Check sheet for the modelled part. Datum: model origin and axes. Units: mm. A direction names the side the tool comes from. Give positions to 0.01 mm unless a question says otherwise; leave off trailing zeros. Loops run counter-clockwise (first coordinate to the right, second up) from the corner with the lowest first, then second, coordinate; pieces in that order, holes last. Notation, with made-up numbers: (89.25, 89) - (147.25, 89) arc R18 cw to (147.25, 113) - close; hole circle Ø2 at (7.25, -39). An arc over 180 degrees is marked (long way). Answer in a Markdown table with one row per item. Add a question column.
(1) Thickness scan on L1, parallel to X at y = 4.5, z = 20; L2, parallel to X at y = 71, z = -13; L3, parallel to X at y = 4, z = -20. Record the ranges inside material, lowest first.
(2) Draft check along X on faces 1 (the face through (-82.21, 2.35, -29.21)), 2 (the face through (-85.24, 89.88, 1.08)), 3 (the face through (76.5, 49, 0)). Enter one of: released by +X, released by -X, zero draft, split by the parting line, or undercut.
(3) Sectioned sample at C-C on z = -20. State how many separate pieces and enclosed holes the cut face has, then the cut area to 3 significant figures.
(4) Sectioned sample at B-B on x = 38. Enter the section's corners in (y, z).
(5) Set-up check for faces 4 (the face through (-76.5, 59, 0)), 5 (the face through (75.62, 8.969, 28.764)), 6 (the face through (76.819, 106.312, -0.623)), 7 (the face through (-78.47, 90.95, 0.78)): record each of +Z, -Z, +X, -X, +Y, -Y from which the full face is reachable in a straight line by a thin tool's end or side.
(6) Go/stop test with flat-tipped pins: P1, Ø5.5, axis at x = 0, z = 20, coming from the -Y side; P2, Ø5, axis at x = -63, z = 19.5, coming from the +Y side; P3, Ø12, axis at y = 85, z = 0, coming from the -X side; P4, Ø1.8, axis at y = 85, z = -15, coming from the +X side. Record where each tip stops, or that it passes through.
(7) Sectioned sample at A-A on y = 44. Enter the section's corners in (x, z).
from build123d import *

# Parameters (mm, degrees)
SKETCH1_W           = 169
SKETCH1_H           = 60
BOSS_EXTRUDE1_DEPTH = 8
SKETCH2_W           = 8
SKETCH2_H           = 60
BOSS_EXTRUDE2_DEPTH = 100
SKETCH3_R           = 10
SKETCH3_R_2         = 1.5
CUT_EXTRUDE1_DEPTH  = 12
SKETCH5_R           = 5
BOSS_EXTRUDE3_DEPTH = 1.5
SKETCH6_R           = 4
CUT_EXTRUDE3_DEPTH  = 15
SKETCH7_R           = 6
CUT_EXTRUDE4_DEPTH  = 4
FILLET1_RADIUS      = 30
FILLET1_LENGTH      = 8
FILLET2_RADIUS      = 30
FILLET2_LENGTH      = 8
FILLET3_R           = 5
FILLET4_R           = 5
FILLET5_R           = 5
FILLET6_R           = 5
CHAMFER1_SIZE       = 2
SKETCH8_R           = 3.1
SKETCH8_R_2         = 3.2
CUT_EXTRUDE5_DEPTH  = 10


with BuildPart() as part:
    # Sketch1 → Boss-Extrude1 (new body)
    with BuildSketch(Plane(origin=(0, 0, 0), x_dir=(1, 0, 0), z_dir=(0, 1, 0))):
        Rectangle(SKETCH1_W, SKETCH1_H)
    extrude(amount=BOSS_EXTRUDE1_DEPTH)

    # Sketch2 → Boss-Extrude2 (add)
    with BuildSketch(Plane(origin=(0, 8, 0), x_dir=(1, 0, 0), z_dir=(0, 1, 0))):
        with Locations((-80.5, 0)):
            Rectangle(SKETCH2_W, SKETCH2_H)
        with Locations((80.5, 0)):
            Rectangle(SKETCH2_W, SKETCH2_H)
    extrude(amount=BOSS_EXTRUDE2_DEPTH)

    # Sketch3 → Cut-Extrude1 (cut)
    with BuildSketch(Plane(origin=(84.5, 0, 0), x_dir=(0, 0, -1), z_dir=(1, 0, 0))):
        with Locations((0, 85)):
            Circle(SKETCH3_R)
        with Locations((0, 70)):
            Circle(SKETCH3_R_2)
        with Locations((0, 100)):
            Circle(SKETCH3_R_2)
        with Locations((-15, 85)):
            Circle(SKETCH3_R_2)
        with Locations((15, 85)):
            Circle(SKETCH3_R_2)
    extrude(amount=-CUT_EXTRUDE1_DEPTH, mode=Mode.SUBTRACT)

    # Sketch5 → Boss-Extrude3 (add)
    with BuildSketch(Plane.ZY.offset(84.5)):
        with Locations(Location((0, 85, 0), (0, 0, 180))):
            Circle(SKETCH5_R)
    extrude(amount=BOSS_EXTRUDE3_DEPTH)

    # Sketch6 → Cut-Extrude3 (cut)
    with BuildSketch(Plane.ZY.offset(86)):
        with Locations((0, 85)):
            Circle(SKETCH6_R)
    extrude(amount=-CUT_EXTRUDE3_DEPTH, mode=Mode.SUBTRACT)

    # Sketch7 → Cut-Extrude4 (cut)
    with BuildSketch(Plane(origin=(-76.5, 0, 0), x_dir=(0, 0, -1), z_dir=(1, 0, 0))):
        with Locations((0, 85)):
            Circle(SKETCH7_R)
    extrude(amount=-CUT_EXTRUDE4_DEPTH, mode=Mode.SUBTRACT)

    # Fillet1: full round fillet: the end face becomes a half cylinder, R = half its width
    fillet1_face = Plane((80.5, 108, 0), x_dir=(-1, 0, 0), z_dir=(0, 1, 0))  # on the end face: x along it, z out of the body
    fillet1_slab = fillet1_face.offset(-FILLET1_RADIUS / 2) * Box(FILLET1_LENGTH, 2 * FILLET1_RADIUS, FILLET1_RADIUS, mode=Mode.PRIVATE)  # the body's end, R deep
    fillet1_round = Plane((80.5, 78, 0), x_dir=(0, 1, 0), z_dir=(-1, 0, 0)) * Cylinder(FILLET1_RADIUS, FILLET1_LENGTH, mode=Mode.PRIVATE)  # its axis R under the face
    add(fillet1_slab - fillet1_round, mode=Mode.SUBTRACT)

    # Fillet2: full round fillet: the end face becomes a half cylinder, R = half its width
    fillet2_face = Plane((-80.5, 108, 0), x_dir=(1, 0, 0), z_dir=(0, 1, 0))  # on the end face: x along it, z out of the body
    fillet2_slab = fillet2_face.offset(-FILLET2_RADIUS / 2) * Box(FILLET2_LENGTH, 2 * FILLET2_RADIUS, FILLET2_RADIUS, mode=Mode.PRIVATE)  # the body's end, R deep
    fillet2_round = Plane((-80.5, 78, 0), x_dir=(0, 1, 0), z_dir=(1, 0, 0)) * Cylinder(FILLET2_RADIUS, FILLET2_LENGTH, mode=Mode.PRIVATE)  # its axis R under the face
    add(fillet2_slab - fillet2_round, mode=Mode.SUBTRACT)

    # Fillet3
    fillet3_edges = [part.edges().sort_by_distance(p)[0] for p in [
        (76.5, 8, 0),
    ]]
    fillet(fillet3_edges, radius=FILLET3_R)

    # Fillet4
    fillet4_edges = [part.edges().sort_by_distance(p)[0] for p in [
        (-76.5, 8, 0),
    ]]
    fillet(fillet4_edges, radius=FILLET4_R)

    # Fillet5
    fillet5_edges = [part.edges().sort_by_distance(p)[0] for p in [
        (84.5, 0, 0),
    ]]
    fillet(fillet5_edges, radius=FILLET5_R)

    # Fillet6
    fillet6_edges = [part.edges().sort_by_distance(p)[0] for p in [
        (-84.5, 0, 0),
    ]]
    fillet(fillet6_edges, radius=FILLET6_R)

    # Chamfer1
    chamfer1_edges = [part.edges().sort_by_distance(p)[0] for p in [
        (75.035533906, 9.464466094, -30),
        (75.035533906, 9.464466094, 30),
        (0, 8, 30),
        (-75.035533906, 9.464466094, 30),
        (-75.035533906, 9.464466094, -30),
        (0, 0, -30),
        (83.035533906, 1.464466094, 30),
        (83.035533906, 1.464466094, -30),
        (0, 0, 30),
        (-83.035533906, 1.464466094, -30),
        (-83.035533906, 1.464466094, 30),
        (76.5, 45.5, -30),
        (84.5, 41.5, -30),
        (84.5, 41.5, 30),
        (76.5, 45.5, 30),
        (76.5, 108, 0),
        (84.5, 108, 0),
        (-84.5, 41.5, -30),
        (-76.5, 45.5, -30),
        (-76.5, 45.5, 30),
        (-84.5, 41.5, 30),
        (-84.5, 108, 0),
        (-76.5, 108, 0),
        (0, 8, -30),
    ]]
    chamfer(chamfer1_edges, length=CHAMFER1_SIZE)

    # Sketch8 → Cut-Extrude5 (cut)
    with BuildSketch(Plane(origin=(0, 8, 0), x_dir=(1, 0, 0), z_dir=(0, 1, 0))):
        with Locations(Location((0, 0, 0), (0, 0, 270))):
            Circle(SKETCH8_R)
        with Locations(Location((0, 20, 0), (0, 0, 270))):
            Circle(SKETCH8_R)
        with Locations(Location((0, -20, 0), (0, 0, 270))):
            Circle(SKETCH8_R)
        with Locations(Location((-20, -20, 0), (0, 0, 270))):
            Circle(SKETCH8_R)
        with Locations(Location((-20, 20, 0), (0, 0, 270))):
            Circle(SKETCH8_R)
        with Locations(Location((-20, 0, 0), (0, 0, 270))):
            Circle(SKETCH8_R)
        with Locations(Location((20, -20, 0), (0, 0, 270))):
            Circle(SKETCH8_R_2)
        with Locations(Location((20, 0, 0), (0, 0, 270))):
            Circle(SKETCH8_R)
        with Locations(Location((20, 20, 0), (0, 0, 270))):
            Circle(SKETCH8_R)
    extrude(amount=-CUT_EXTRUDE5_DEPTH, mode=Mode.SUBTRACT)


solid = part.part
Reply:
| question | item | result |
|---|---|---|
| 1 | L1 | -84.47 to -23.1, -16.9 to -3.1, 3.1 to 16.8, 23.2 to 84.47 |
| 1 | L2 | -84.5 to -76.5, 76.5 to 84.5 |
| 1 | L3 | -84.4 to -23.1, -16.9 to -3.1, 3.1 to 16.9, 23.1 to 84.4 |
| 2 | face 1 | released by -X |
| 2 | face 2 | zero draft |
| 2 | face 3 | undercut |
| 3 | separate pieces | 4 |
| 3 | enclosed holes | 0 |
| 3 | area | 2,670 mm^2 |
| 4 | outline | (0, -28) - (2, -30) - (6, -30) - (8, -28) - (8, 28) - (6, 30) - (2, 30) - (0, 28) - close |
| 5 | face 4 | +Z, -Z, +Y |
| 5 | face 5 | +Z, +Y |
| 5 | face 6 | +Y |
| 5 | face 7 | +X |
| 6 | P1 | through |
| 6 | P2 | y = 8 |
| 6 | P3 | x = -86 |
| 6 | P4 | x = -76.5 |
| 7 | outline | (-84.5, -28) - (-82.5, -30) - (-78.5, -30) - (-76.5, -28) - (-76.5, 28) - (-78.5, 30) - (-82.5, 30) - (-84.5, 28) - close; (76.5, -28) - (78.5, -30) - (82.5, -30) - (84.5, -28) - (84.5, 28) - (82.5, 30) - (78.5, 30) - (76.5, 28) - close |
